For this review, take the finished solid that the model builds, in its own axes (mm). Face numbers are marked on the shaded views. Coordinates: 2 decimals unless noted, no trailing zeros. Write each loop counter-clockwise with the first axis right and the second up, starting at its lowest first coordinate (ties: lowest second). Pieces come first, ordered by that corner, then holes. Notation, with made-up numbers: (12, 53.5) - (29, 53.5) arc R26 cw to (29, 81.5) - close; hole circle Ø6 at (-10, 46.5). An arc over 180 degrees is marked (long way). Use one line per item in the form item = value. Start each with the question number.
1) Insertion check: P1, Ø3, axis at y = 27, z = 1.5, coming from the -X side; P2, Ø1, axis at y = -23.5, z = 1.5, coming from the -X side; P3, Ø4, axis at x = -64, z = 1, coming from the -Y side. Each pin has a flat end and moves straight along its axis. Give the tip position at first contact, or say it passes through.
2) For L1, parallel to Y at x = 0, z = 1.25; L2, parallel to X at y = 1, z = 2.5; L3, parallel to X at y = -57, z = 0.5, list the stretches that pass through material, from the lowest coordinate up. Write a range as from..to.
3) Mouldability with a two-part tool opening along Y and no side actions: class the marked faces 1 and 2 as pulls with the +Y half, pulls with the -Y half, needs draft (parallel to the pull), parting line crosses it, or undercut.
4) We need section B-B (y = 0). Give the boundary of the cut face in (x, z), plus the area to 3 significant figures.
5) We need section D-D (y = 50). Give the boundary of the cut face in (x, z).
6) We need section C-C (x = 0). Give the boundary of the cut face in (y, z).
```python
from build123d import *

# Parameters (mm, degrees)
F0_R     = 59.56666
F1_DEPTH = 3.81
F2_R     = 38.83477
F3_DEPTH = 25.4
F4_W     = 12.7
F4_H     = 38.1
F4_W_2   = 38.1
F4_H_2   = 12.7
F5_DEPTH = 3.81


with BuildPart() as f1:
    # F0 (on Top) → F1 (new body, symmetric)
    with BuildSketch(Plane.XY):
        Circle(F0_R)
    extrude(amount=F1_DEPTH, both=True)

    # F2 (on face) → F3 (cut)
    with BuildSketch(Plane.XY.offset(3.81)):
        Circle(F2_R)
    extrude(amount=-F3_DEPTH, mode=Mode.SUBTRACT)

    # F4 (on Top) → F5 (join, symmetric)
    with BuildSketch(Plane.XY):
        Polygon((-51.550063, -25.89613), (-60.530319, -34.876386), (-33.589551, -61.817154), (-24.609294, -52.836898), align=None)
        Polygon((26.389541, -51.384653), (36.118306, -59.548056), (60.608514, -30.361762), (50.879749, -22.19836), align=None)
        with Locations((60.338904, 0.166861)):
            Rectangle(F4_W, F4_H)
        with Locations((0.23175, -59.773433)):
            Rectangle(F4_W_2, F4_H_2)
        with Locations((-61.395693, 1.594452)):
            Rectangle(F4_W, F4_H)
        Polygon((-60.575688, 35.438669), (-51.595432, 26.458413), (-24.654663, 53.399182), (-33.63492, 62.379438), align=None)
        with Locations((0.23175, 61.052699)):
            Rectangle(F4_W_2, F4_H_2)
        Polygon((34.518826, 60.477025), (25.53857, 51.496769), (52.479338, 24.556001), (61.459594, 33.536257), align=None)
    extrude(amount=F5_DEPTH, both=True)


solid = f1.part
```
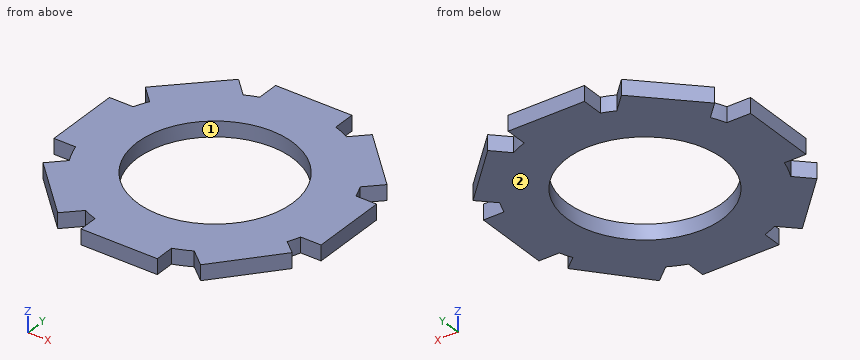
Determined:
q1.P1 = -53.83
q1.P2 = -54.95
q1.P3 = -17.46
q2.L1 = -66.12..-38.83, 38.83..67.4
q2.L2 = -67.75..-38.82, 38.82..66.69
q2.L3 = -38.41..-28.77, -18.82..19.28, 33.08..38.26
q3.face_1 = undercut
q3.face_2 = needs draft
q4.outline = (-67.75, -3.81) - (-38.83, -3.81) - (-38.83, 3.81) - (-67.75, 3.81) - close; (38.83, -3.81) - (66.69, -3.81) - (66.69, 3.81) - (38.83, 3.81) - close
q4.area = 433 mm²
q5.outline = (-46.01, -3.81) - (45, -3.81) - (45, 3.81) - (-46.01, 3.81) - close
q6.outline = (-66.12, -3.81) - (-38.83, -3.81) - (-38.83, 3.81) - (-66.12, 3.81) - close; (38.83, -3.81) - (67.4, -3.81) - (67.4, 3.81) - (38.83, 3.81) - close
